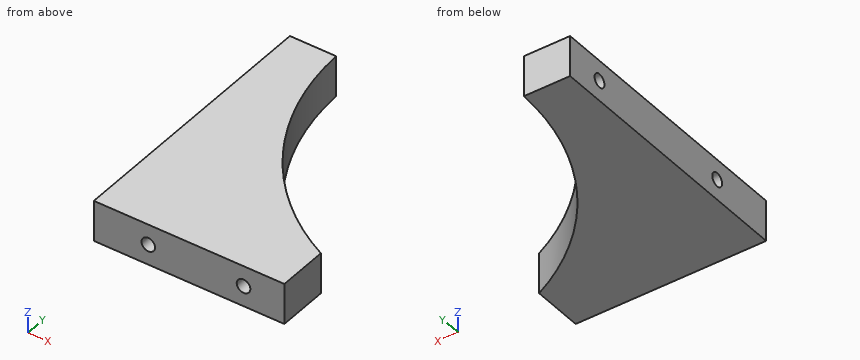
from build123d import *

# Parameters (mm, degrees)
BOSS_EXTRU_1_DEPTH      = 15
ESQUISSE7_R             = 2.5
ENL_V_MAT_EXTRU_4_DEPTH = 16
ESQUISSE5_R             = 2.5
ENL_V_MAT_EXTRU_5_DEPTH = 16
ESQUISSE8_R             = 2.5
ENL_V_MAT_EXTRU_6_DEPTH = 16
ESQUISSE9_R             = 2.5
ENL_V_MAT_EXTRU_7_DEPTH = 16
ENL_V_START             = -3
ESQUISSE10_W            = 11
ESQUISSE10_H            = 6.5
ESQUISSE10_W_2          = 9.5
ESQUISSE10_H_2          = 14.5
ENL_V_MAT_EXTRU_8_DEPTH = 9


with BuildPart() as part:
    # Esquisse1 → Boss.-Extru.1 (new body)
    with BuildSketch(Plane.XY):
        with BuildLine():
            Line((0, 100), (17, 100))
            ThreePointArc((17, 100), (32.078733461, 51.873825012), (70, 18.625148861))
            Line((70, 18.625148861), (70, 0))
            Line((70, 0), (0, 0))
            Line((0, 0), (0, 100))
        make_face()
    extrude(amount=BOSS_EXTRU_1_DEPTH)

    # Esquisse7 → Enlèv. mat.-Extru.4 (cut)
    with BuildSketch(Plane.ZY):
        with Locations((7.5, 25)):
            Circle(ESQUISSE7_R)
    extrude(amount=-ENL_V_MAT_EXTRU_4_DEPTH, mode=Mode.SUBTRACT)

    # Esquisse5 → Enlèv. mat.-Extru.5 (cut)
    with BuildSketch(Plane.ZY):
        with Locations((7.5, 85)):
            Circle(ESQUISSE5_R)
    extrude(amount=-ENL_V_MAT_EXTRU_5_DEPTH, mode=Mode.SUBTRACT)

    # Esquisse8 → Enlèv. mat.-Extru.6 (cut)
    with BuildSketch(Plane.XZ):
        with Locations(Location((20, 7.5, 0), (0, 0, 270))):
            Circle(ESQUISSE8_R)
    extrude(amount=-ENL_V_MAT_EXTRU_6_DEPTH, mode=Mode.SUBTRACT)

    # Esquisse9 → Enlèv. mat.-Extru.7 (cut)
    with BuildSketch(Plane.XZ):
        with Locations(Location((55, 7.5, 0), (0, 0, 270))):
            Circle(ESQUISSE9_R)
    extrude(amount=-ENL_V_MAT_EXTRU_7_DEPTH, mode=Mode.SUBTRACT)

    # Esquisse10 → Enlèv. mat.-Extru.8 (cut)
    with BuildSketch(Plane.XY.offset(15).offset(ENL_V_START)):
        with BuildLine():
            Line((3, 79.5), (15.014172538, 79.5))
            ThreePointArc((15.014172538, 79.5), (26.862682219, 51.335667796), (47.020836751, 28.373403185))
            Line((47.020836751, 28.373403185), (47.020836751, 22.591228546))
            Line((47.020836751, 22.591228546), (47.020836751, 18.330678811))
            Line((47.020836751, 18.330678811), (47.020836751, 3))
            Line((47.020836751, 3), (25.5, 3))
            Line((25.5, 3), (25.5, 14.739450265))
            Line((25.5, 14.739450265), (25.5, 19))
            Line((25.5, 19), (19, 19))
            Line((19, 19), (19, 30.5))
            Line((19, 30.5), (3, 30.5))
            Line((3, 30.5), (3, 79.5))
        make_face()
        with Locations((8.5, 93.75)):
            Rectangle(ESQUISSE10_W, ESQUISSE10_H)
        with Locations((8.75, 11.25)):
            Rectangle(ESQUISSE10_W_2, ESQUISSE10_H_2)
    extrude(amount=-ENL_V_MAT_EXTRU_8_DEPTH, mode=Mode.SUBTRACT)


solid = part.part
Here's how the part is built. I have some questions about the finished solid (model axes, mm). Coordinates: 2 decimals unless noted, no trailing zeros. Order: outer loops, then holes, each group sorted by start corner. A loop starts at its lowest first (then second) coordinate and runs counter-clockwise, first axis right, second up. Notation, with made-up numbers: M -29.75,-36.75 L 9.25,-36.75 A7 ccw 9.25,-28.75 Z; hole C 19.25,75.25 d11. An arc over 180 degrees is marked long. Answer as CSV lines item,"result".
Item 1: Imagine slicing it at B-B on y = 10.5. Write out the boundary of the cut face in (x, z), plus the area to 3 significant figures.
Results found:
outline,"M 0,0 L 70,0 L 70,15 L 0,15 Z; hole M 4,3 L 13.5,3 L 13.5,12 L 4,12 Z; hole C 20,7.5 d5; hole M 25.5,3 L 47.02,3 L 47.02,12 L 25.5,12 Z; hole C 55,7.5 d5"
area,"732 mm2"
Item 2: Imagine slicing it at A-A on x = 8. Write out the boundary of the cut face in (y, z).
Results found:
outline,"M 0,0 L 100,0 L 100,15 L 0,15 Z; hole M 4,3 L 18.5,3 L 18.5,12 L 4,12 Z; hole C 25,7.5 d5; hole M 30.5,3 L 79.5,3 L 79.5,12 L 30.5,12 Z; hole C 85,7.5 d5; hole M 90.5,3 L 97,3 L 97,12 L 90.5,12 Z"
Item 3: For pin 1 (1.5 mm diameter, centred on y = 21, z = 11.5, fed in from +X); pin 2 (1 mm diameter, centred on y = 83, z = 6, fed in from +X); pin 3 (5 mm diameter, centred on y = 94.5, z = 9.5, fed in from +X), each with a flat end and sliding along its axis, tell me the tip position at first contact or that it passes through.
Results found:
pin 1,"x = 66.77"
pin 2,"x = 19.19"
pin 3,"x = 17.58"
Item 4: If I drill on line 1 (Y direction, x = 7.5, z = 11); line 2 (X direction, y = 5, z = 7.5); line 3 (Y direction, x = 11.25, z = 7.5), over which ranges is the centre line in solid material (lowest first)?
Results found:
line 1,"0 to 4, 18.5 to 30.5, 79.5 to 90.5, 97 to 100"
line 2,"0 to 4, 13.5 to 17.5, 22.5 to 25.5, 47.02 to 52.5, 57.5 to 70"
line 3,"0 to 4, 18.5 to 22.5, 27.5 to 30.5, 79.5 to 82.5, 87.5 to 90.5, 97 to 100"
Item 5: Imagine slicing it at D-D on y = 78. Write out the boundary of the cut face in (x, z).
Results found:
outline,"M 0,0 L 20.31,0 L 20.31,15 L 0,15 Z; hole M 3,3 L 15.39,3 L 15.39,12 L 3,12 Z"
Item 6: Imagine slicing it at C-C on x = 41.5. Write out the boundary of the cut face in (y, z), plus the area to 3 significant figures.
Results found:
outline,"M 0,0 L 39.73,0 L 39.73,15 L 0,15 Z; hole M 3,3 L 33.29,3 L 33.29,12 L 3,12 Z"
area,"323 mm2"
